Geometry check sheet. Reference: the model listing, model coordinates, mm. Face numbers are marked on the shaded views. A direction names the side the tool comes from. Coordinates: 2 decimals unless noted, no trailing zeros. Write each loop counter-clockwise with the first axis right and the second up, starting at its lowest first coordinate (ties: lowest second). Pieces come first, ordered by that corner, then holes.
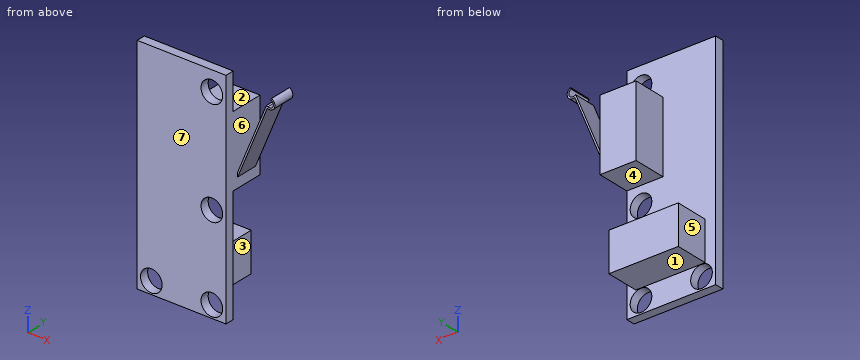
from build123d import *

# Parameters (mm, degrees)
SKETCH1_W           = 16
SKETCH1_H           = 40
BOSS_EXTRUDE1_DEPTH = 1.6
SKETCH2_R           = 1.95
CUT_EXTRUDE1_DEPTH  = 1.6
SKETCH3_W           = 12.5
SKETCH3_H           = 7
SKETCH3_W_2         = 6.5
SKETCH3_H_2         = 12.8
BOSS_EXTRUDE2_DEPTH = 6
BOSS_EXTRUDE3_START = 1
BOSS_EXTRUDE3_DEPTH = 4


with BuildPart() as part:
    # Sketch1 → Boss-Extrude1 (new body)
    with BuildSketch(Plane(origin=(0, 0, 0), x_dir=(1, 0, 0), z_dir=(0, 1, 0))):
        with Locations((8, 20)):
            Rectangle(SKETCH1_W, SKETCH1_H)
    extrude(amount=BOSS_EXTRUDE1_DEPTH)

    # Sketch2 → Cut-Extrude1 (cut)
    with BuildSketch(Plane(origin=(0, 1.6, 0), x_dir=(1, 0, 0), z_dir=(0, 1, 0))):
        with Locations(Location((2.55, 37.792201536, 0), (0, 0, 270))):
            Circle(SKETCH2_R)
        with Locations(Location((13.45, 37.792201536, 0), (0, 0, 270))):
            Circle(SKETCH2_R)
        with Locations(Location((13.45, 3.55, 0), (0, 0, 270))):
            Circle(SKETCH2_R)
        with Locations(Location((13.45, 22.55, 0), (0, 0, 270))):
            Circle(SKETCH2_R)
    extrude(amount=-CUT_EXTRUDE1_DEPTH, mode=Mode.SUBTRACT)

    # Sketch3 → Boss-Extrude2 (add)
    with BuildSketch(Plane(origin=(0, 1.6, 0), x_dir=(1, 0, 0), z_dir=(0, 1, 0))):
        with Locations((8.15, 32.3)):
            Rectangle(SKETCH3_W, SKETCH3_H)
        with Locations((12.75, 12.9)):
            Rectangle(SKETCH3_W_2, SKETCH3_H_2)
    extrude(amount=BOSS_EXTRUDE2_DEPTH)

    # Sketch4 → Boss-Extrude3 (add)
    with BuildSketch(Plane(origin=(0.760107299, 7.6, -17.342959561), x_dir=(1, 0, 0), z_dir=(0, -1, 0)).offset(BOSS_EXTRUDE3_START)):
        with BuildLine():
            Line((15.239892701, -0.157040439), (20.579395829, 12.784740982))
            ThreePointArc((20.579395829, 12.784740982), (21.885201868, 13.32776086), (21.34218199, 14.633566899))
            Line((21.34218199, 14.633566899), (21.227764066, 14.356243012))
            ThreePointArc((21.227764066, 14.356243012), (21.60787798, 13.442178784), (20.693813753, 13.06206487))
            Line((20.693813753, 13.06206487), (20.416533297, 13.176588062))
            Line((20.416533297, 13.176588062), (15.239892701, 0.629549605))
            Line((15.239892701, 0.629549605), (15.239892701, -0.157040439))
        make_face()
    extrude(amount=BOSS_EXTRUDE3_DEPTH)


solid = part.part
1. Access from +Z, -Z, +X, -X, +Y, -Y to the whole of each face (thin tool, end or side, straight path). Record for the marked faces 1, 2, 3 and 4.
Computed values:
face 1: -Z, +X, -X, +Y
face 2: +Z, -X, +Y
face 3: -Z, +X, +Y
face 4: +X, -X, +Y
2. Thickness scan on line 1 along Z through (x, y) = (14.75, 1.5); line 2 along X through (y, z) = (0.85, -22.55); line 3 along X through (y, z) = (5, -35). Record the ranges inside material, lowest first.
Computed values:
line 1: z = -40 to -39.25, -36.34 to -24, -21.1 to -5, -2.1 to 0
line 2: x = 0 to 11.5, 15.4 to 16
line 3: x = 1.9 to 14.4
3. Gauge pin test, flat ends, axial feed: pin 1 Ø6 at (x, z) = (2.55, -37.79) entering from -Y; pin 2 Ø4 at (x, z) = (2.5, -9) entering from +Y; pin 3 Ø1.8 at (x, y) = (5, 3.5) entering from -Z; pin 4 Ø4 at (x, z) = (19.5, -5.5) entering from +Y. Record the tip position at first contact, or that the pin passes through.
Computed values:
pin 1: stops at y = 0
pin 2: stops at y = 1.6
pin 3: stops at z = -35.8
pin 4: stops at y = 6.6
4. Sectioned sample at D-D, the plane y = 6. Record the boundary of the cut face in (x, z).
Computed values:
outline: (1.9, -35.8) - (14.4, -35.8) - (14.4, -28.8) - (1.9, -28.8) - close; (9.5, -19.3) - (16, -19.3) - (16, -17.5) - (21.34, -4.56) arc R1 ccw to (22.1, -2.71) - (21.99, -2.99) arc R0.7 cw to (21.45, -4.28) - (21.18, -4.17) - (16, -16.71) - (16, -6.5) - (9.5, -6.5) - close
5. Sectioned sample at B-B, the plane x = 2.55. Record the boundary of the cut face in (y, z).
Computed values:
outline: (0, -40) - (1.6, -40) - (1.6, -39.74) - (0, -39.74) - close; (0, -35.84) - (1.6, -35.84) - (1.6, -35.8) - (7.6, -35.8) - (7.6, -28.8) - (1.6, -28.8) - (1.6, 0) - (0, 0) - close
6. Sectioned sample at A-A, the plane y = 0.75. Record the boundary of the cut face in (x, z).
Computed values:
outline: (0, -40) - (16, -40) - (16, 0) - (0, 0) - close; hole circle Ø3.9 at (2.55, -37.79); hole circle Ø3.9 at (13.45, -37.79); hole circle Ø3.9 at (13.45, -22.55); hole circle Ø3.9 at (13.45, -3.55)
7. Draft check along X on the marked faces 5, 6 and 7. Enter one of: released by +X, released by -X, zero draft, split by the parting line, or undercut.
Computed values:
face 5: released by -X
face 6: undercut
face 7: zero draft
8. Sectioned sample at C-C, the plane z = -22.55. Record the boundary of the cut face in (x, y).
Computed values:
outline: (0, 0) - (11.5, 0) - (11.5, 1.6) - (0, 1.6) - close; (15.4, 0) - (16, 0) - (16, 1.6) - (15.4, 1.6) - close
